Input: dimensioned drawing with shaded views. Units: mm. Origin: part minimum x, y, z. A direction names the side the tool comes from. Give positions to 0.01 mm unless a question says otherwise; leave off trailing zeros. Write each loop counter-clockwise with the first axis right and the second up, starting at its lowest first coordinate (ties: lowest second). Pieces come first, ordered by that corner, then holes. Notation, with made-up numbers: M 19.5,83.5 L 29.5,83.5 A13 ccw 29.5,87.5 Z; hole C 8,-9 d6. An arc over 180 degrees is marked long. Use CSV: the item, a comma, the result in double quotes. Start each with the question number.
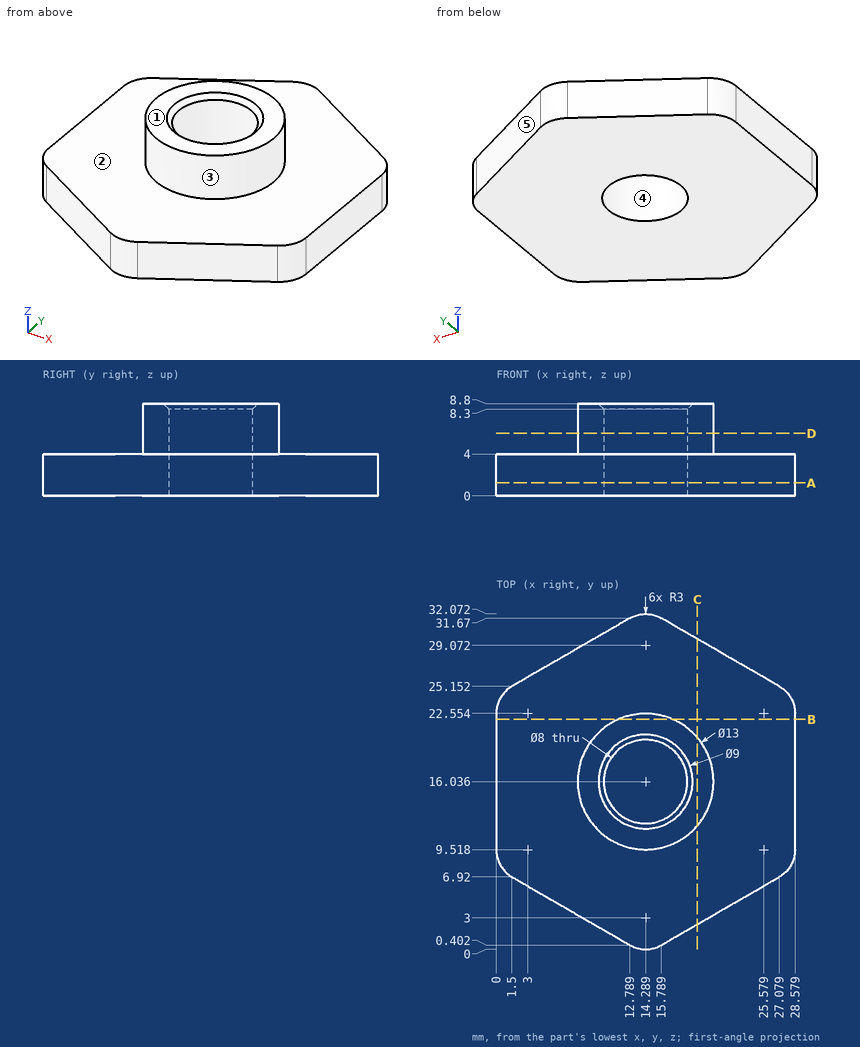
Q1. First-contact query: pin 1 Ø1 at (x, y) = (21, 24) entering from +Z; pin 2 Ø4 at (y, z) = (13, 6.5) entering from -X; pin 3 Ø2 at (x, z) = (13, 4) entering from -Y. Flat tips, straight axial feed; report the tip coordinate or a pass-through.
Q2. Section D-D, the plane z = 6. Return the cut outline in (x, y).
Q3. Set-up query: the marked faces 1 and 2. Return all of +Z, -Z, +X, -X, +Y, -Y with unobstructed straight access to the full face (end or side cutting, diameter ignored); none if empty.
Q4. Material intervals for L1, parallel to Z at x = 18.5, y = 8.5; L2, parallel to Y at x = 12.75, z = 2.75 (1 decimal); L3, parallel to X at y = 15, z = 0.5 (1 decimal), sorted ascending. Write a range as [from, to].
Q5. Section A-A, the plane z = 1.25. Return the cut outline in (x, y), and give its area (3 significant figures).
Q6. Pull-direction query (X, two-part tool) for the marked faces 3, 4 and 5; classes: released by +X, released by -X, zero draft, split by the parting line, or undercut.
Q7. Section C-C, the plane x = 19.25. Return the cut outline in (y, z) (1 decimal), and give its area (3 significant figures).
Q8. Section B-B, the plane y = 22. Return the cut outline in (x, z) (1 decimal), and give its area (3 significant figures).
Check result:
1,pin 1,"stops at z = 4"
1,pin 2,"stops at x = 7.87"
1,pin 3,"stops at y = 0.01"
2,outline,"C 14.29,16.04 d13; hole C 14.29,16.04 d8"
3,face 1,"+Z, +X, -X, +Y, -Y"
3,face 2,"+Z"
4,L1,"z = [0, 4]"
4,L2,"y = [0.4, 12.3], [19.7, 31.6]"
4,L3,"x = [0, 10.4], [18.2, 28.6]"
5,outline,"M 0,9.52 A3 ccw 1.5,6.92 L 12.79,0.4 A3 ccw 15.79,0.4 L 27.08,6.92 A3 ccw 28.58,9.52 L 28.58,22.55 A3 ccw 27.08,25.15 L 15.79,31.67 A3 ccw 12.79,31.67 L 1.5,25.15 A3 ccw 0,22.55 Z; hole C 14.29,16.04 d8"
5,area,"654 mm²"
6,face 3,"split by the parting line"
6,face 4,"undercut"
6,face 5,"released by +X"
7,outline,"M 2.4,0 L 29.7,0 L 29.7,4 L 20.2,4 L 20.2,8.8 L 11.8,8.8 L 11.8,4 L 2.4,4 Z"
7,area,"149 mm²"
8,outline,"M 0,0 L 28.6,0 L 28.6,4 L 16.9,4 L 16.9,8.8 L 11.7,8.8 L 11.7,4 L 0,4 Z"
8,area,"139 mm²"
